from build123d import *

# Parameters (mm, degrees)
SKETCH1_W               = 61.1
SKETCH1_H               = 60
BOSS_EXTRUDE1_DEPTH     = 5
BOSS_EXTRUDE2_DEPTH     = 24
MIRROR2_COPY_1_DEPTH    = 24
CUT_EXTRUDE1_START      = -47.739758236
SKETCH3_R               = 1.75
CUT_EXTRUDE1_DEPTH      = 54.785521216
MIRROR4_START           = -47.739758236
MIRROR4_COPY_1_SKETCH_R = 1.75
MIRROR4_COPY_1_DEPTH    = 54.785521216
MIRROR5_START           = -47.739758236
MIRROR5_COPY_1_SKETCH_R = 1.75
MIRROR5_COPY_1_DEPTH    = 54.785521216
MIRROR5_COPY_2_SKETCH_R = 1.75
MIRROR5_COPY_2_DEPTH    = 54.785521216
MIRROR5_COPY_3_SKETCH_R = 1.75
MIRROR5_COPY_3_DEPTH    = 54.785521216
SKETCH9_W               = 6
SKETCH9_H               = 2.5
BOSS_EXTRUDE4_DEPTH     = 8
SKETCH9_3_W             = 6
SKETCH9_3_H             = 2.5
CUT_EXTRUDE7_DEPTH      = 10
MIRROR7_COPY_1_SKETCH_W = 6
MIRROR7_COPY_1_SKETCH_H = 2.5
MIRROR7_COPY_1_DEPTH    = 8
MIRROR7_COPY_2_SKETCH_W = 6
MIRROR7_COPY_2_SKETCH_H = 2.5
MIRROR7_COPY_2_DEPTH    = 10
SKETCH10_R              = 1.55
CUT_EXTRUDE8_DEPTH      = 10
SKETCH11_R              = 1.55
CUT_EXTRUDE9_DEPTH      = 10


with BuildPart() as part:
    # Sketch1 → Boss-Extrude1 (new body)
    with BuildSketch(Plane(origin=(0, 0, 0), x_dir=(1, 0, 0), z_dir=(0, 1, 0))):
        Rectangle(SKETCH1_W, SKETCH1_H)
    extrude(amount=BOSS_EXTRUDE1_DEPTH)

    # Sketch2 → Boss-Extrude2 (add)
    with BuildSketch(Plane.XY.offset(30)):
        with BuildLine():
            Line((-30.55, 13.55), (-30.55, 5))
            Line((-30.55, 5), (-13.45, 5))
            Line((-13.45, 5), (-13.45, 13.55))
            Line((-13.45, 13.55), (-14.45, 13.55))
            ThreePointArc((-14.45, 13.55), (-22, 6), (-29.55, 13.55))
            Line((-29.55, 13.55), (-30.55, 13.55))
        make_face()
    boss_extrude2 = extrude(amount=-BOSS_EXTRUDE2_DEPTH)

    # Mirror1: Boss-Extrude2 across plane
    add(boss_extrude2.mirror(Plane.XY))

    # Mirror2: Boss-Extrude2 across plane
    add(boss_extrude2.mirror(Plane(origin=(0, 0, 0), x_dir=(0, 0, 1), z_dir=(1, 0, 0))))

    # Mirror2 copy 1 sketch → Mirror2 copy 1 (add)
    with BuildSketch(Plane(origin=(0, 0, -30), x_dir=(-1, 0, 0), z_dir=(0, 0, -1))):
        with BuildLine():
            Line((-30.55, 13.55), (-30.55, 5))
            Line((-30.55, 5), (-13.45, 5))
            Line((-13.45, 5), (-13.45, 13.55))
            Line((-13.45, 13.55), (-14.45, 13.55))
            ThreePointArc((-14.45, 13.55), (-22, 6), (-29.55, 13.55))
            Line((-29.55, 13.55), (-30.55, 13.55))
        make_face()
    extrude(amount=-MIRROR2_COPY_1_DEPTH)

    # Sketch3 → Cut-Extrude1 (cut)
    with BuildSketch(Plane(origin=(-17.775, 17.775, 0), x_dir=(0.707106781, 0.707106781, 0), z_dir=(-0.707106781, 0.707106781, 0)).offset(CUT_EXTRUDE1_START)):
        with Locations(Location((-15.52081528, -18, 0), (0, 0, 180))):  # turned: the seam where the file's is
            Circle(SKETCH3_R)
    cut_extrude1 = extrude(amount=CUT_EXTRUDE1_DEPTH, mode=Mode.SUBTRACT)

    # Mirror3: Cut-Extrude1 across plane
    add(cut_extrude1.mirror(Plane.ZY.offset(22)), mode=Mode.SUBTRACT)

    # Mirror4: Cut-Extrude1 across plane
    add(cut_extrude1.mirror(Plane.XY), mode=Mode.SUBTRACT)

    # Mirror4 copy 1 sketch → Mirror4 copy 1 (cut)
    with BuildSketch(Plane(origin=(-26.225, 17.775, 0), x_dir=(-0.707106781, 0.707106781, 0), z_dir=(0.707106781, 0.707106781, 0)).offset(MIRROR4_START)):
        with Locations(Location((-15.52081528, -18, 0), (0, 0, 180))):  # turned: the seam where the file's is
            Circle(MIRROR4_COPY_1_SKETCH_R)
    extrude(amount=MIRROR4_COPY_1_DEPTH, mode=Mode.SUBTRACT)

    # Mirror5: Cut-Extrude1 across plane
    add(cut_extrude1.mirror(Plane(origin=(0, 0, 0), x_dir=(0, 0, 1), z_dir=(1, 0, 0))), mode=Mode.SUBTRACT)

    # Mirror5 copy 1 sketch → Mirror5 copy 1 (cut)
    with BuildSketch(Plane(origin=(17.775, 17.775, 0), x_dir=(-0.707106781, 0.707106781, 0), z_dir=(0.707106781, 0.707106781, 0)).offset(MIRROR5_START)):
        with Locations(Location((-15.52081528, -18, 0), (0, 0, 180))):  # turned: the seam where the file's is
            Circle(MIRROR5_COPY_1_SKETCH_R)
    extrude(amount=MIRROR5_COPY_1_DEPTH, mode=Mode.SUBTRACT)

    # Mirror5 copy 2 sketch → Mirror5 copy 2 (cut)
    with BuildSketch(Plane(origin=(26.225, 17.775, 0), x_dir=(0.707106781, 0.707106781, 0), z_dir=(-0.707106781, 0.707106781, 0)).offset(MIRROR5_START)):
        with Locations((-15.52081528, 18)):
            Circle(MIRROR5_COPY_2_SKETCH_R)
    extrude(amount=MIRROR5_COPY_2_DEPTH, mode=Mode.SUBTRACT)

    # Mirror5 copy 3 sketch → Mirror5 copy 3 (cut)
    with BuildSketch(Plane(origin=(26.225, 17.775, 0), x_dir=(0.707106781, 0.707106781, 0), z_dir=(-0.707106781, 0.707106781, 0)).offset(MIRROR5_START)):
        with Locations(Location((-15.52081528, -18, 0), (0, 0, 180))):  # turned: the seam where the file's is
            Circle(MIRROR5_COPY_3_SKETCH_R)
    extrude(amount=MIRROR5_COPY_3_DEPTH, mode=Mode.SUBTRACT)

    # Sketch9 → Boss-Extrude4 (add)
    with BuildSketch(Plane.XY.offset(30)):
        Polygon((-13.45, 7.8), (-13.45, 5), (-9.45, 5), (-9.45, 5.3), (-3.45, 5.3), (-3.45, 5), (-1.45, 5), (-1.45, 7.8), align=None)
        with Locations((-6.45, 3.75)):
            Rectangle(SKETCH9_W, SKETCH9_H)
    boss_extrude4 = extrude(amount=-BOSS_EXTRUDE4_DEPTH)

    # Sketch9_3 → Cut-Extrude7 (cut)
    with BuildSketch(Plane.XY.offset(30)):
        with Locations((-6.45, 3.75)):
            Rectangle(SKETCH9_3_W, SKETCH9_3_H)
    cut_extrude7 = extrude(amount=-CUT_EXTRUDE7_DEPTH, mode=Mode.SUBTRACT)

    # Mirror6: Boss-Extrude4, Cut-Extrude7 across plane
    add(boss_extrude4.mirror(Plane.XY))
    add(cut_extrude7.mirror(Plane.XY), mode=Mode.SUBTRACT)

    # Mirror7: Boss-Extrude4, Cut-Extrude7 across plane
    add(boss_extrude4.mirror(Plane(origin=(0, 0, 0), x_dir=(0, 0, 1), z_dir=(1, 0, 0))))
    add(cut_extrude7.mirror(Plane(origin=(0, 0, 0), x_dir=(0, 0, 1), z_dir=(1, 0, 0))), mode=Mode.SUBTRACT)

    # Mirror7 copy 1 sketch → Mirror7 copy 1 (add)
    with BuildSketch(Plane(origin=(0, 0, -30), x_dir=(-1, 0, 0), z_dir=(0, 0, -1))):
        Polygon((-13.45, 7.8), (-13.45, 5), (-9.45, 5), (-9.45, 5.3), (-3.45, 5.3), (-3.45, 5), (-1.45, 5), (-1.45, 7.8), align=None)
        with Locations((-6.45, 3.75)):
            Rectangle(MIRROR7_COPY_1_SKETCH_W, MIRROR7_COPY_1_SKETCH_H)
    extrude(amount=-MIRROR7_COPY_1_DEPTH)

    # Mirror7 copy 2 sketch → Mirror7 copy 2 (cut)
    with BuildSketch(Plane(origin=(0, 0, -30), x_dir=(-1, 0, 0), z_dir=(0, 0, -1))):
        with Locations((-6.45, 3.75)):
            Rectangle(MIRROR7_COPY_2_SKETCH_W, MIRROR7_COPY_2_SKETCH_H)
    extrude(amount=-MIRROR7_COPY_2_DEPTH, mode=Mode.SUBTRACT)

    # Sketch10 → Cut-Extrude8 (cut)
    with BuildSketch(Plane(origin=(0, 7.8, 0), x_dir=(1, 0, 0), z_dir=(0, 1, 0))):
        with Locations(Location((-6.45, 26, 0), (0, 0, 270))):  # turned: the seam where the file's is
            Circle(SKETCH10_R)
        with Locations(Location((6.45, 26, 0), (0, 0, 270))):  # turned: the seam where the file's is
            Circle(SKETCH10_R)
        with Locations(Location((6.45, -26, 0), (0, 0, 270))):  # turned: the seam where the file's is
            Circle(SKETCH10_R)
        with Locations(Location((-6.45, -26, 0), (0, 0, 270))):  # turned: the seam where the file's is
            Circle(SKETCH10_R)
    extrude(amount=-CUT_EXTRUDE8_DEPTH, mode=Mode.SUBTRACT)

    # Sketch11 → Cut-Extrude9 (cut)
    with BuildSketch(Plane.XZ):
        with Locations(Location((0, 10, 0), (0, 0, 270))):  # turned: the seam where the file's is
            Circle(SKETCH11_R)
        with Locations(Location((0, -10, 0), (0, 0, 270))):  # turned: the seam where the file's is
            Circle(SKETCH11_R)
    extrude(amount=-CUT_EXTRUDE9_DEPTH, mode=Mode.SUBTRACT)


solid = part.part
Part model, mm, in its own coordinate system. A direction names the side the tool comes from. Give positions to 0.01 mm unless a question says otherwise; leave off trailing zeros. Loops run counter-clockwise (first coordinate to the right, second up) from the corner with the lowest first, then second, coordinate; pieces in that order, holes last.
(1) Pin check, flat tips, straight feed: pin 1 (4 mm diameter, centred on x = -6.45, z = -26, fed in from +Y); pin 2 (4 mm diameter, centred on x = 6.45, z = -26, fed in from -Y); pin 3 (10 mm diameter, centred on x = 5.5, z = 12, fed in from +Y). Stop position of each tip, or through.
Return value:
pin 1: stops at y = 7.8
pin 2: stops at y = 0
pin 3: stops at y = 5
(2) 3-axis set-ups, long thin cutter, end or side, ignore diameter. For faces 3 (the flat face through (-6, 2.5, 24)), 4 (the flat face through (22.1, 5.5, 6)), 5 (the flat face through (-1.45, 6, 26)): which of +Z, -Z, +X, -X, +Y, -Y reach the whole face in a straight line?
Return value:
face 3: +Z
face 4: +X, -X, +Y
face 5: +Z, -Z, +Y
(3) Drill centre lines: line 1 along X through (y, z) = (3.5, 20.5); line 2 along Y through (x, z) = (5, -24.5); line 3 along X through (y, z) = (5.75, 7). Where is each one in solid material? Low to high.
Return value:
line 1: x = -30.55 to -9.45, -3.45 to 3.45, 9.45 to 30.55
line 2: y = 0 to 2.5, 5.3 to 7.8
line 3: x = -30.55 to -13.45, 13.45 to 30.55
(4) Band-saw the part on A-A (z = -10). Write the cut outline in (x, y), and give its area (3 significant figures).
Return value:
outline: (-30.55, 0) - (-1.55, 0) - (-1.55, 5) - (-13.45, 5) - (-13.45, 13.55) - (-14.45, 13.55) arc R7.55 cw to (-29.55, 13.55) - (-30.55, 13.55) - close; (1.55, 0) - (30.55, 0) - (30.55, 13.55) - (29.55, 13.55) arc R7.55 cw to (14.45, 13.55) - (13.45, 13.55) - (13.45, 5) - (1.55, 5) - close
area: 403 mm2
(5) Pull direction Y, two halves, no side cores. Call faces 1 (the flat face through (-8, 5.3, 27)), 2 (the flat face through (13.45, 9, -16)): pulls with the +Y half, pulls with the -Y half, needs draft (parallel to the pull), parting line crosses it, or undercut.
Return value:
face 1: undercut
face 2: needs draft
(6) Band-saw the part on B-B (x = -6.45). Count the separate pieces of the cut face and the enclosed holes in it, and give its area (3 significant figures).
Return value:
separate pieces: 7
enclosed holes: 0
area: 259 mm2
